from build123d import *

# Parameters (mm, degrees)
ESQUISSE1_W             = 80
ESQUISSE1_H             = 3
BOSS_EXTRU_1_DEPTH      = 338
ESQUISSE3_W             = 8
ESQUISSE3_H             = 3
BOSS_EXTRU_2_DEPTH      = 6
ESQUISSE4_W             = 8
ESQUISSE4_H             = 6
ENL_V_MAT_EXTRU_2_DEPTH = 6
ESQUISSE5_W             = 3
ESQUISSE5_H             = 30
ENL_V_MAT_EXTRU_3_DEPTH = 3


with BuildPart() as part:
    # Esquisse1 → Boss.-Extru.1 (new body)
    with BuildSketch(Plane.XY):
        with Locations((40, 1.5)):
            Rectangle(ESQUISSE1_W, ESQUISSE1_H)
    extrude(amount=BOSS_EXTRU_1_DEPTH)

    # Esquisse3 → Boss.-Extru.2 (add)
    with BuildSketch(Plane(origin=(0, 0, 0), x_dir=(-1, 0, 0), z_dir=(0, 0, -1))):
        with Locations((-10, 1.5)):
            Rectangle(ESQUISSE3_W, ESQUISSE3_H)
        with Locations((-30, 1.5)):
            Rectangle(ESQUISSE3_W, ESQUISSE3_H)
        with Locations((-50, 1.5)):
            Rectangle(ESQUISSE3_W, ESQUISSE3_H)
        with Locations((-70, 1.5)):
            Rectangle(ESQUISSE3_W, ESQUISSE3_H)
    boss_extru_2 = extrude(amount=BOSS_EXTRU_2_DEPTH)

    # Symétrie1: Boss.-Extru.2 across plane
    add(boss_extru_2.mirror(Plane(origin=(0, 0, 169), x_dir=(1, 0, 0), z_dir=(0, 0, -1))))

    # Esquisse4 → Enlèv. mat.-Extru.2 (cut)
    with BuildSketch(Plane.XZ):
        with Locations((10, -3)):
            Rectangle(ESQUISSE4_W, ESQUISSE4_H)
    extrude(amount=-ENL_V_MAT_EXTRU_2_DEPTH, mode=Mode.SUBTRACT)

    # Esquisse5 → Enlèv. mat.-Extru.3 (cut)
    with BuildSketch(Plane.XZ):
        with Locations((73.5, 129)):
            Rectangle(ESQUISSE5_W, ESQUISSE5_H)
    extrude(amount=-ENL_V_MAT_EXTRU_3_DEPTH, mode=Mode.SUBTRACT)


solid = part.part
Geometry check sheet. Reference: the model listing, model coordinates, mm. Give positions to 0.01 mm unless a question says otherwise; leave off trailing zeros. Loops run counter-clockwise (first coordinate to the right, second up) from the corner with the lowest first, then second, coordinate; pieces in that order, holes last.
(1) Thickness scan on L1, parallel to X at y = 2.4, z = 143; L2, parallel to Z at x = 65.5, y = 0.3; L3, parallel to Z at x = 10.5, y = 2.5. Record the ranges inside material, lowest first.
From the geometry:
L1: x = 0 to 72, 75 to 80
L2: z = 0 to 338
L3: z = 0 to 344
(2) Depth check by flat-ended pin: pin 1 Ø1.5 at (x, y) = (40.5, 1) entering from -Z; pin 2 Ø1.5 at (y, z) = (2, 342.5) entering from -X; pin 3 Ø1.5 at (x, y) = (23, 1) entering from +Z. Enter the tip coordinate at first touch or a pass-through.
From the geometry:
pin 1: stops at z = 0
pin 2: stops at x = 6
pin 3: stops at z = 338
(3) Section check A-A on z = 130. Record the cut outline in (x, y).
From the geometry:
outline: (0, 0) - (72, 0) - (72, 3) - (0, 3) - close; (75, 0) - (80, 0) - (80, 3) - (75, 3) - close
(4) Section check B-B on x = 40.5. Record the cut outline in (y, z).
From the geometry:
outline: (0, 0) - (3, 0) - (3, 338) - (0, 338) - close
